from build123d import *

# Parameters (mm, degrees)
F1_DEPTH = 63.5
F2_DEPTH = 25.4
F0_W     = 25.4
F0_H     = 19.05
F3_DEPTH = 25.4
F4_DEPTH = 7.9375


with BuildPart() as f1:
    # F0 (on Front) → F1 (new body, symmetric)
    with BuildSketch(Plane.XZ):
        Polygon((22.225, 9.525), (-41.275, 9.525), (-41.275, -9.525), (41.275, -9.525), (41.275, 9.525), align=None)
    extrude(amount=F1_DEPTH, both=True)

    # F0 (on Front) → F2 (join, symmetric)
    with BuildSketch(Plane.XZ):
        with BuildLine():
            Line((22.225, 28.1995688956), (22.225, 9.525))
            Line((22.225, 9.525), (41.275, 9.525))
            Line((41.275, 9.525), (41.275, 28.1995688956))
            ThreePointArc((41.275, 28.1995688956), (43.9569999969, 37.0290862051), (51.0967796432, 42.8752))
            Line((51.0967796432, 42.8752), (60.325, 42.8752))
            Line((60.325, 42.8752), (60.325, 61.9252))
            Line((60.325, 61.9252), (48.076002446, 61.9252))
            ThreePointArc((48.076002446, 61.9252), (29.431188792, 49.4462893534), (22.225, 28.1995688956))
        make_face()
    extrude(amount=F2_DEPTH, both=True)

    # F0 (on Front) → F3 (join, symmetric)
    with BuildSketch(Plane.XZ):
        with Locations((73.025, 52.4002)):
            Rectangle(F0_W, F0_H)
    extrude(amount=F3_DEPTH, both=True)

    # F0 (on Front) → F4 (join, symmetric)
    with BuildSketch(Plane.XZ):
        with BuildLine():
            add(Edge.make_bspline(
                [(-41.275, 9.525), (-32.5510911644, 38.347762078), (0, 61.8160702288), (48.076002446, 61.9252)],
                knots=[0, 0, 0, 0, 103.5827331081, 103.5827331081, 103.5827331081, 103.5827331081], degree=3))
            Line((-41.275, 9.525), (22.225, 9.525))
            Line((22.225, 9.525), (22.225, 28.1995688956))
            ThreePointArc((22.225, 28.1995688956), (29.431188792, 49.4462893534), (48.076002446, 61.9252))
        make_face()
    extrude(amount=F4_DEPTH, both=True)

    # F0 (on Front) → F5 (revolve)
    with BuildSketch(Plane.XZ):
        Polygon((85.725, 66.675), (85.725, 61.9252), (85.725, 42.8752), (85.725, 38.1), (111.125, 38.1), (111.125, 66.675), align=None)
    revolve(axis=Axis((85.725, 0, 52.3875), (0, 0, 1)))


solid = f1.part
Check sheet for the modelled part. Datum: model origin and axes. Units: mm. A direction names the side the tool comes from. Round coordinates to 2 decimals unless told otherwise and drop trailing zeros. Loops run counter-clockwise (first coordinate to the right, second up) from the corner with the lowest first, then second, coordinate; pieces in that order, holes last.
1. Set-up check for faces 1 (the flat face through (22.225, -17, 19)), 2 (the flat face through (46, -25.4, 42)), 3 (the flat face through (86, 0, 38.1)), 4 (the cylindrical face through (29.63, 16.55, 49.7)): record each of +Z, -Z, +X, -X, +Y, -Y from which the full face is reachable in a straight line by a thin tool's end or side.
2. Sectioned sample at A-A on z = 5.5. Record the boundary of the cut face in (x, y) (3 decimals), and give its area (3 significant figures).
3. Scan lines: probe 1 along Z at (x, y) = (79.5, 22.5) (3 decimals); probe 2 along Y at (x, z) = (71, 43.5); probe 3 along X at (y, z) = (-20, 17.5) (3 decimals). Record each from-to range of solid material in increasing order.
4. Sectioned sample at B-B on y = -53. Record the boundary of the cut face in (x, z) (3 decimals), and give its area (3 significant figures).
5. Gauge pin test, flat ends, axial feed: pin 1 Ø15 at (x, y) = (93, 4) entering from -Z; pin 2 Ø5 at (y, z) = (16, 22.5) entering from -X (3 decimals); pin 3 Ø15.5 at (x, z) = (14, 38.5) entering from -Y. Record the tip position at first contact, or that the pin passes through.
Recorded:
1. face 1: +Z, -X, -Y
1. face 2: +Z, +X, -X, -Y
1. face 3: -Z, +X, +Y, -Y
1. face 4: +Z, -X, +Y
2. outline: (-41.275, -63.5) - (41.275, -63.5) - (41.275, 63.5) - (-41.275, 63.5) - close
2. area: 10,500 mm2
3. probe 1: z = 38.1 to 66.675
3. probe 2: y = -25.4 to 25.4
3. probe 3: x = 22.225 to 41.275
4. outline: (-41.275, -9.525) - (41.275, -9.525) - (41.275, 9.525) - (-41.275, 9.525) - close
4. area: 1,570 mm2
5. pin 1: stops at z = 38.1
5. pin 2: stops at x = 22.225
5. pin 3: stops at y = -7.94
